Study the drawing (mm; zero at the part's minimum x, y, z) and answer. Give positions to 0.01 mm unless a question says otherwise; leave off trailing zeros. Loops run counter-clockwise (first coordinate to the right, second up) from the corner with the lowest first, then second, coordinate; pieces in that order, holes last. Notation, with made-up numbers: (74, 68.25) - (114, 68.25) arc R20 cw to (114, 88.25) - close; hole circle Ø3 at (80, 86.25). An arc over 180 degrees is marked (long way). Write item = value, one per line. Start each with the question number.
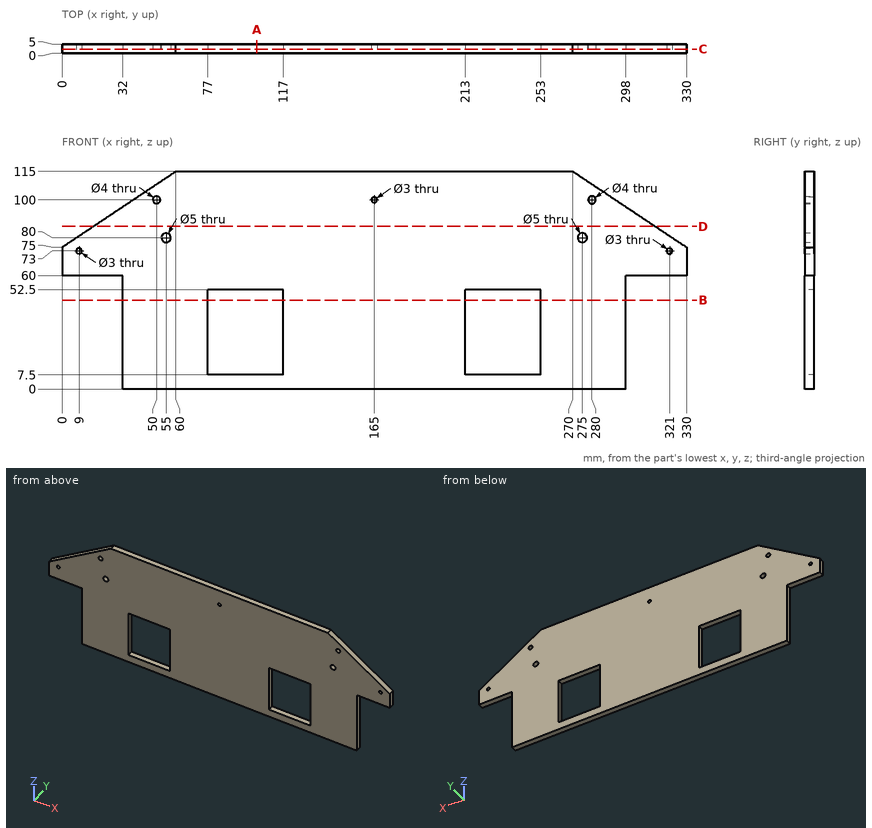
1. A cutting plane is placed at A-A on x = 103. Give the vertices of the cut face in (y, z), and give its area (3 significant figures).
2. Given P1, Ø1.5, axis at y = 4, z = 96.5, coming from the -X side (3 decimals); P2, Ø2.5, axis at y = 2.5, z = 19.5, coming from the -X side; P3, Ø4.5, axis at x = 55, z = 80, coming from the -Y side; P4, Ø1.5, axis at y = 2, z = 41, coming from the +X side, each flat-ended and moving along its own axis, determine where each tip first touches the part or whether it passes through.
3. A cutting plane is placed at D-D on z = 86. Give the vertices of the cut face in (x, y).
4. A cutting plane is placed at B-B on z = 47. Give the vertices of the cut face in (x, y).
5. Consider line 1 along X through (y, z) = (3.8, 30.5); line 2 along X through (y, z) = (2.85, 80); line 3 along X through (y, z) = (4.3, 100.5). Determine where each line is inside the solid, lowest interval first. Write a range as [from, to].
6. A cutting plane is placed at C-C on y = 2.35. Give the number of separate pieces and of enclosed holes in the cut face, and give its area (3 significant figures).
Reply:
q1.outline = (0, 0) - (5, 0) - (5, 7.5) - (0, 7.5) - close; (0, 52.5) - (5, 52.5) - (5, 115) - (0, 115) - close
q1.area = 350 mm^2
q2.P1 = 31.125
q2.P2 = 32
q2.P3 = through
q2.P4 = 298
q3.outline = (16.5, 0) - (313.5, 0) - (313.5, 5) - (16.5, 5) - close
q4.outline = (32, 0) - (77, 0) - (77, 5) - (32, 5) - close; (117, 0) - (213, 0) - (213, 5) - (117, 5) - close; (253, 0) - (298, 0) - (298, 5) - (253, 5) - close
q5.line_1 = [32, 77], [117, 213], [253, 298]
q5.line_2 = [7.5, 52.5], [57.5, 272.5], [277.5, 322.5]
q5.line_3 = [38.25, 48.06], [51.94, 163.59], [166.41, 278.06], [281.94, 291.75]
q6.separate_pieces = 1
q6.enclosed_holes = 9
q6.area = 28,000 mm^2
